from build123d import *

# Parameters (mm, degrees)
F0_W     = 49.5
F0_H     = 31
F0_W_2   = 45.5
F0_H_2   = 27
F1_DEPTH = 15
F2_W     = 23
F2_H     = 8
F3_DEPTH = 31.001
F4_R     = 1
F5_R     = 0.5
F6_W     = 49.5
F6_H     = 1.5
F7_DEPTH = 15
F8_W     = 49.5
F8_H     = 5.7
F9_DEPTH = 2
F10_R    = 0.5
F11_SIZE = 1


with BuildPart() as f1:
    # F0 (on Front) → F1 (new body)
    with BuildSketch(Plane.XZ):
        Rectangle(F0_W, F0_H)
        Rectangle(F0_W_2, F0_H_2, mode=Mode.SUBTRACT)
    extrude(amount=F1_DEPTH)

    # F2 (on face) → F3 (cut, through all)
    with BuildSketch(Plane.XY.offset(15.5)):
        with Locations((0, -9)):
            Rectangle(F2_W, F2_H)
    extrude(amount=-F3_DEPTH, mode=Mode.SUBTRACT)

    # F4
    f4_edges = [f1.edges().sort_by_distance(p)[0] for p in [
        (24.75, -7.5, 15.5),
        (24.75, -7.5, -15.5),
        (-24.75, -7.5, 15.5),
        (-24.75, -7.5, -15.5),
    ]]
    fillet(f4_edges, radius=F4_R)

    # F5
    f5_edges = [f1.edges().sort_by_distance(p)[0] for p in [
        (-22.75, -7.5, 13.5),
        (22.75, -7.5, 13.5),
        (22.75, -7.5, -13.5),
        (-22.75, -7.5, -13.5),
    ]]
    fillet(f5_edges, radius=F5_R)



with BuildPart() as f7:
    # F6 (on Front) → F7 (new body, through all)
    with BuildSketch(Plane.XZ):
        with Locations((0, -18.45)):
            Rectangle(F6_W, F6_H)
    extrude(amount=F7_DEPTH)


with BuildPart() as f1_1:
    add(f1.part)

    add(f7.part)  # F9 merges F7
    # F8 (on Front) → F9 (join)
    with BuildSketch(Plane.XZ):
        with Locations((0, -16.35)):
            Rectangle(F8_W, F8_H)
    extrude(amount=F9_DEPTH)

    # F10
    f10_edges = [f1_1.edges().sort_by_distance(p)[0] for p in [
        (24.75, -7.5, -19.2),
        (24.75, -8.5, -17.7),
        (-24.75, -7.5, -19.2),
        (-24.75, -8.5, -17.7),
    ]]
    fillet(f10_edges, radius=F10_R)

    # F11
    f11_edges = [f1_1.edges().sort_by_distance(p)[0] for p in [
        (0, -15, 13.5),
    ]]
    chamfer(f11_edges, length=F11_SIZE)


solid = f1_1.part
Design review of the part built by this model. Coordinates are the model's own, in mm. A direction names the side the tool comes from. Coordinates: 2 decimals unless noted, no trailing zeros. Loops run counter-clockwise (first coordinate to the right, second up) from the corner with the lowest first, then second, coordinate; pieces in that order, holes last. Notation, with made-up numbers: (54.5, -16.75) - (95.5, -16.75) arc R22 cw to (95.5, 7.25) - close; hole circle Ø3 at (77, 80.5). An arc over 180 degrees is marked (long way). Use CSV: the item, a comma, the result in double quotes. Start each with the question number.
1. Add section C-C on z = 4. Give the boundary of the cut face in (x, y).
2. For faces 4 (the flat face through (0, -5, -14)), 5 (the cylindrical face through (-24.465, -8.591, -15.199)), 6 (the cylindrical face through (24.449, -8.591, -15.215)), 7 (the conical face through (22.954, -14.507, 13.72)), 8 (the flat face through (0, -4, -15.5)), list the 3-axis set-ups (+Z, -Z, +X, -X, +Y, -Y) from which the entire face can be reached by the end or side of a thin tool; tool diameter is ignored.
3. Add section A-A on x = -21.5. Give the boundary of the cut face in (y, z), plus the area to 3 significant figures.
4. Add section D-D on x = -9. Give the boundary of the cut face in (y, z).
5. Mouldability with a two-part tool opening along Y and no side actions: class faces 1 (the conical face through (22.97, -14.507, -13.704)), 2 (the flat face through (0, -13, 15)), 3 (the flat face through (0, -4, -13.5)) as released by +Y, released by -Y, zero draft, split by the parting line, or undercut.
6. Clearance check with flat-ended pins moving along their axes: pin 1 (1 mm diameter, centred on x = 0.5, z = -14.5, fed in from +Y); pin 2 (0.6 mm diameter, centred on y = -9, z = -15, fed in from -X); pin 3 (2 mm diameter, centred on x = 1.5, y = -9.5, fed in from +Z); pin 4 (1.1 mm diameter, centred on x = -6.5, z = -16.5, fed in from -Y). State where each tip first meets the part, or that it passes through.
7. Add section B-B on y = -3.5. Give the boundary of the cut face in (x, z), plus the area to 3 significant figures.
8. To check wall thickness, follow probe 1 along Z at (x, y) = (19, -13.75); probe 2 along X at (y, z) = (-8, 11); probe 3 along Y at (x, z) = (17, -17). State the ranges of each line that lie inside material, in increasing order.
Resolved:
1,outline,"(-24.75, -15) - (-23.75, -15) - (-22.75, -14) - (-22.75, 0) - (-24.75, 0) - close; (22.75, -14) - (23.75, -15) - (24.75, -15) - (24.75, 0) - (22.75, 0) - close"
2,face 4,"+Z"
2,face 5,"-X, -Y"
2,face 6,"+X, -Y"
2,face 7,"-Y"
2,face 8,"+X, -X, -Y"
3,outline,"(-15, -19.2) - (0, -19.2) - (0, -13.5) - (-14, -13.5) - (-15, -14.5) - (-15, -15.5) - (-2, -15.5) - (-2, -17.7) - (-15, -17.7) - close; (-15, 14.5) - (-14, 13.5) - (0, 13.5) - (0, 15.5) - (-15, 15.5) - close"
3,area,"85.9 mm2"
4,outline,"(-15, -19.2) - (0, -19.2) - (0, -13.5) - (-5, -13.5) - (-5, -15.5) - (-2, -15.5) - (-2, -17.7) - (-15, -17.7) - close; (-15, -15.5) - (-13, -15.5) - (-13, -13.5) - (-14, -13.5) - (-15, -14.5) - close; (-15, 14.5) - (-14, 13.5) - (-13, 13.5) - (-13, 15.5) - (-15, 15.5) - close; (-5, 13.5) - (0, 13.5) - (0, 15.5) - (-5, 15.5) - close"
5,face 1,"released by -Y"
5,face 2,"undercut"
5,face 3,"zero draft"
6,pin 1,"y = 0"
6,pin 2,"x = -24.73"
6,pin 3,"z = -17.7"
6,pin 4,"y = -2"
7,outline,"(-24.75, -18.7) arc R0.5 ccw to (-24.25, -19.2) - (24.25, -19.2) arc R0.5 ccw to (24.75, -18.7) - (24.75, -18.2) arc R0.5 ccw to (24.25, -17.7) - (-24.25, -17.7) arc R0.5 ccw to (-24.75, -18.2) - close; (-24.75, -14.5) arc R1 ccw to (-23.75, -15.5) - (23.75, -15.5) arc R1 ccw to (24.75, -14.5) - (24.75, 14.5) arc R1 ccw to (23.75, 15.5) - (-23.75, 15.5) arc R1 ccw to (-24.75, 14.5) - close; hole (-22.75, -13) arc R0.5 ccw to (-22.25, -13.5) - (22.25, -13.5) arc R0.5 ccw to (22.75, -13) - (22.75, 13) arc R0.5 ccw to (22.25, 13.5) - (-22.25, 13.5) arc R0.5 ccw to (-22.75, 13) - close"
7,area,"379 mm2"
8,probe 1,"-19.2 to -17.7, -15.5 to -13.5, 13.5 to 15.5"
8,probe 2,"-24.75 to -22.75, 22.75 to 24.75"
8,probe 3,"-2 to 0"
